The model under review builds one solid part; all positions refer to its coordinate system, in mm. Coordinates: 2 decimals unless noted, no trailing zeros. Loops run counter-clockwise (first coordinate to the right, second up) from the corner with the lowest first, then second, coordinate; pieces in that order, holes last. Notation, with made-up numbers: (-12, 17) - (-1, 17) arc R15 ccw to (-1, 32) - close; hole circle Ø4 at (41, -4). An arc over 180 degrees is marked (long way). Answer in a Markdown table with one row per item. Add a question column.
(1) We need section A-A on y = 50. Give the number of separate pieces and of enclosed holes in the cut face, plus the area to 3 significant figures.
(2) For line 1 along Z through (x, y) = (136, 95), list the stretches that pass through material, from the lowest coordinate up.
(3) For P1, Ø15.5, axis at x = -63, z = -0.5, coming from the +Y side, flat-tipped, find the tip position at first contact; note if it passes through.
(4) We need section C-C on y = -150. Write out the cut boundary in (x, z).
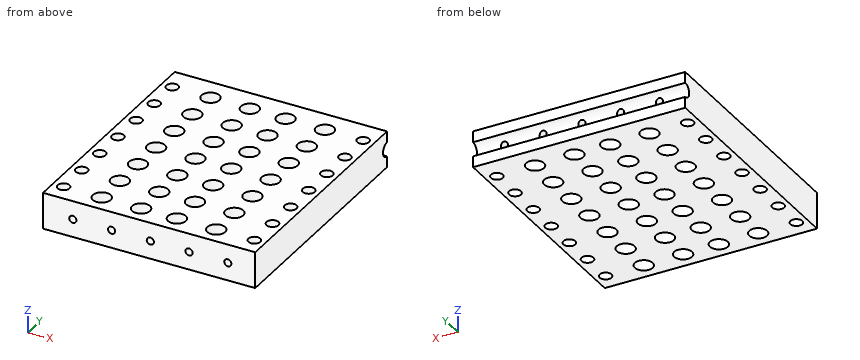
from build123d import *

# Parameters (mm, degrees)
SKETCH1_W           = 356
SKETCH1_H           = 400
BOSS_EXTRUDE1_DEPTH = 30.5
SKETCH4_R           = 10
SKETCH4_R_2         = 6
BOSS_EXTRUDE2_DEPTH = 400
CUT_EXTRUDE1_DEPTH  = 357
SKETCH4_2_R         = 6
CUT_EXTRUDE2_DEPTH  = 401
SKETCH4_3_R         = 6
CUT_EXTRUDE3_DEPTH  = 401.0000001
SKETCH8_R           = 15
SKETCH8_R_2         = 10
CUT_EXTRUDE4_DEPTH  = 62


with BuildPart() as part:
    # Sketch1 → Boss-Extrude1 (new body, symmetric)
    with BuildSketch(Plane.XY):
        Rectangle(SKETCH1_W, SKETCH1_H)
    extrude(amount=BOSS_EXTRUDE1_DEPTH, both=True)

    # Sketch4 → Boss-Extrude2 (add, through all)
    with BuildSketch(Plane(origin=(0, 200, 0), x_dir=(1, 0, 0), z_dir=(0, 1, 0))):
        with Locations((-128, 0.5)):
            Circle(SKETCH4_R)
        with Locations((-128, 0.5)):
            Circle(SKETCH4_R_2, mode=Mode.SUBTRACT)
        with Locations((-63, 0.5)):
            Circle(SKETCH4_R)
        with Locations((-63, 0.5)):
            Circle(SKETCH4_R_2, mode=Mode.SUBTRACT)
        with Locations((2, 0.5)):
            Circle(SKETCH4_R)
        with Locations((2, 0.5)):
            Circle(SKETCH4_R_2, mode=Mode.SUBTRACT)
        with Locations((67, 0.5)):
            Circle(SKETCH4_R)
        with Locations((67, 0.5)):
            Circle(SKETCH4_R_2, mode=Mode.SUBTRACT)
        with Locations((132, 0.5)):
            Circle(SKETCH4_R)
        with Locations((132, 0.5)):
            Circle(SKETCH4_R_2, mode=Mode.SUBTRACT)
    extrude(amount=-BOSS_EXTRUDE2_DEPTH)

    # Sketch6 → Cut-Extrude1 (cut, through all)
    with BuildSketch(Plane(origin=(178, 0, 0), x_dir=(0, 0, -1), z_dir=(1, 0, 0))):
        with BuildLine():
            Line((-12, 200), (12, 200))
            ThreePointArc((12, 200), (0, 188), (-12, 200))
        make_face()
    extrude(amount=-CUT_EXTRUDE1_DEPTH, mode=Mode.SUBTRACT)

    # Sketch4<2> → Cut-Extrude2 (cut, through all)
    with BuildSketch(Plane(origin=(0, 200, 0), x_dir=(1, 0, 0), z_dir=(0, 1, 0))):
        with Locations((-128, 0.5)):
            Circle(SKETCH4_2_R)
    extrude(amount=-CUT_EXTRUDE2_DEPTH, mode=Mode.SUBTRACT)

    # Sketch4<3> → Cut-Extrude3 (cut, through all)
    with BuildSketch(Plane(origin=(0, 200, 0), x_dir=(1, 0, 0), z_dir=(0, 1, 0))):
        with Locations((-128, 0.5)):
            Circle(SKETCH4_3_R)
        with Locations((-63, 0.5)):
            Circle(SKETCH4_3_R)
        with Locations((2, 0.5)):
            Circle(SKETCH4_3_R)
        with Locations((67, 0.5)):
            Circle(SKETCH4_3_R)
        with Locations((132, 0.5)):
            Circle(SKETCH4_3_R)
    extrude(amount=-CUT_EXTRUDE3_DEPTH, mode=Mode.SUBTRACT)

    # Sketch8 → Cut-Extrude4 (cut, through all)
    with BuildSketch(Plane.XY.offset(30.5)):
        with Locations((-30, 160)):
            Circle(SKETCH8_R)
        with Locations((-30, 105)):
            Circle(SKETCH8_R)
        with Locations((-30, 50)):
            Circle(SKETCH8_R)
        with Locations((-30, -5)):
            Circle(SKETCH8_R)
        with Locations((-30, -60)):
            Circle(SKETCH8_R)
        with Locations((-30, -115)):
            Circle(SKETCH8_R)
        with Locations((-30, -170)):
            Circle(SKETCH8_R)
        with Locations((30, -170)):
            Circle(SKETCH8_R)
        with Locations((30, -115)):
            Circle(SKETCH8_R)
        with Locations((30, -60)):
            Circle(SKETCH8_R)
        with Locations((30, -5)):
            Circle(SKETCH8_R)
        with Locations((30, 50)):
            Circle(SKETCH8_R)
        with Locations((30, 105)):
            Circle(SKETCH8_R)
        with Locations((30, 160)):
            Circle(SKETCH8_R)
        with Locations((-96, -170)):
            Circle(SKETCH8_R)
        with Locations((-96, -115)):
            Circle(SKETCH8_R)
        with Locations((-96, -60)):
            Circle(SKETCH8_R)
        with Locations((-96, -5)):
            Circle(SKETCH8_R)
        with Locations((-96, 50)):
            Circle(SKETCH8_R)
        with Locations((-96, 105)):
            Circle(SKETCH8_R)
        with Locations((-96, 160)):
            Circle(SKETCH8_R)
        with Locations((96, 160)):
            Circle(SKETCH8_R)
        with Locations((96, 105)):
            Circle(SKETCH8_R)
        with Locations((96, 50)):
            Circle(SKETCH8_R)
        with Locations((96, -5)):
            Circle(SKETCH8_R)
        with Locations((96, -60)):
            Circle(SKETCH8_R)
        with Locations((96, -115)):
            Circle(SKETCH8_R)
        with Locations((96, -170)):
            Circle(SKETCH8_R)
        with Locations((-160, 160)):
            Circle(SKETCH8_R_2)
        with Locations((-160, 105)):
            Circle(SKETCH8_R_2)
        with Locations((-160, 50)):
            Circle(SKETCH8_R_2)
        with Locations((-160, -5)):
            Circle(SKETCH8_R_2)
        with Locations((-160, -60)):
            Circle(SKETCH8_R_2)
        with Locations((-160, -115)):
            Circle(SKETCH8_R_2)
        with Locations((-160, -170)):
            Circle(SKETCH8_R_2)
        with Locations((160, -170)):
            Circle(SKETCH8_R_2)
        with Locations((160, -115)):
            Circle(SKETCH8_R_2)
        with Locations((160, -60)):
            Circle(SKETCH8_R_2)
        with Locations((160, -5)):
            Circle(SKETCH8_R_2)
        with Locations((160, 50)):
            Circle(SKETCH8_R_2)
        with Locations((160, 105)):
            Circle(SKETCH8_R_2)
        with Locations((160, 160)):
            Circle(SKETCH8_R_2)
    extrude(amount=-CUT_EXTRUDE4_DEPTH, mode=Mode.SUBTRACT)


solid = part.part
Outcome:
| question | item | result |
|---|---|---|
| 1 | separate pieces | 7 |
| 1 | enclosed holes | 5 |
| 1 | area | 11,400 mm² |
| 2 | line 1 | -30.5 to -4.97, 3.97 to 30.5 |
| 3 | P1 | y = 191.29 |
| 4 | outline | (-178, -30.5) - (178, -30.5) - (178, 30.5) - (-178, 30.5) - close; hole circle Ø12 at (-128, -0.5); hole circle Ø12 at (-63, -0.5); hole circle Ø12 at (2, -0.5); hole circle Ø12 at (67, -0.5); hole circle Ø12 at (132, -0.5) |
